For this review, take the finished solid that the model builds, in its own axes (mm). Face numbers are marked on the shaded views. Give positions to 0.01 mm unless a question says otherwise; leave off trailing zeros. Loops run counter-clockwise (first coordinate to the right, second up) from the corner with the lowest first, then second, coordinate; pieces in that order, holes last.
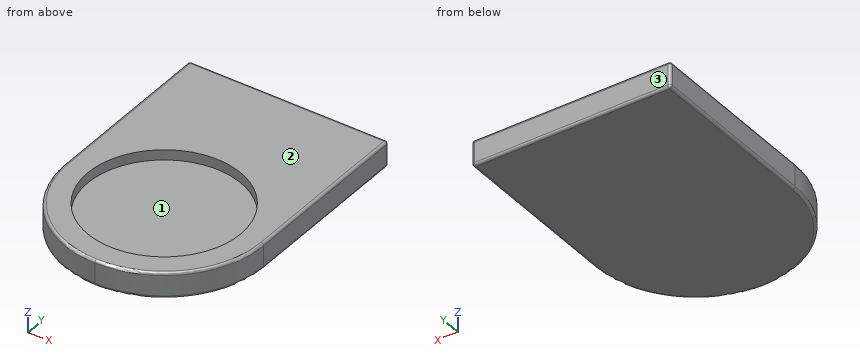
```python
from build123d import *

# Parameters (mm, degrees)
F1_DEPTH = 12.7
F2_DEPTH = 7.62
F3_R     = 1.27


with BuildPart() as f1:
    # F0 (on Top) → F1 (new body)
    with BuildSketch(Plane.XY):
        with BuildLine():
            Line((-49.53, 88.9), (-49.53, 0))
            ThreePointArc((-49.53, 0), (-35.0229988722, -35.0229988722), (0, -49.53))
            Line((0, -49.53), (0, -38.1))
            ThreePointArc((0, -38.1), (-38.1, 0), (0, 38.1))
            Line((0, 38.1), (0, 88.9))
            Line((0, 88.9), (-49.53, 88.9))
        make_face()
        with BuildLine():
            Line((0, -38.1), (0, -49.53))
            ThreePointArc((0, -49.53), (35.0229988722, -35.0229988722), (49.53, 0))
            Line((49.53, 0), (49.53, 88.9))
            Line((49.53, 88.9), (0, 88.9))
            Line((0, 88.9), (0, 38.1))
            ThreePointArc((0, 38.1), (26.9407683632, 26.9407683632), (38.1, 0))
            ThreePointArc((38.1, 0), (26.9407683632, -26.9407683632), (0, -38.1))
        make_face()
    extrude(amount=F1_DEPTH)

    # F0 (on Top) → F2 (join)
    with BuildSketch(Plane.XY):
        with BuildLine():
            ThreePointArc((0, 38.1), (-38.1, 0), (0, -38.1))
            Line((0, -38.1), (0, 38.1))
        make_face()
        with BuildLine():
            Line((0, 38.1), (0, -38.1))
            ThreePointArc((0, -38.1), (26.9407683632, -26.9407683632), (38.1, 0))
            ThreePointArc((38.1, 0), (26.9407683632, 26.9407683632), (0, 38.1))
        make_face()
    extrude(amount=F2_DEPTH)

    # F3
    f3_edges = [f1.edges().sort_by_distance(p)[0] for p in [
        (49.53, 44.45, 12.7),
        (49.53, 88.9, 6.35),
        (0, 88.9, 12.7),
        (0, 88.9, 0),
        (49.53, 44.45, 0),
        (-49.53, 88.9, 6.35),
    ]]
    fillet(f3_edges, radius=F3_R)


solid = f1.part
```
Q1. Consider section A-A on z = 9. Give the boundary of the cut face in (x, y).
Answers:
outline: (-49.53, 0) arc R49.53 ccw to (49.53, 0) - (49.53, 87.63) arc R1.27 ccw to (48.26, 88.9) - (-48.26, 88.9) arc R1.27 ccw to (-49.53, 87.63) - close; hole circle Ø76.2 at (0, 0)
Q2. For pin 1 Ø1 at (y, z) = (-28, 3) entering from -X; pin 2 Ø23 at (x, y) = (4.5, 0.5) entering from +Z; pin 3 Ø1 at (x, z) = (-29, 9) entering from -Y, all flat-tipped, find the tip position at first contact; note any pin that passes through.
Answers:
pin 1: stops at x = -41.19
pin 2: stops at z = 7.62
pin 3: stops at y = -40.51
Q3. Consider section B-B on y = 26. Give the boundary of the cut face in (x, z), plus the area to 3 significant figures.
Answers:
outline: (-49.53, 1.27) arc R1.27 ccw to (-48.26, 0) - (48.26, 0) arc R1.27 ccw to (49.53, 1.27) - (49.53, 11.43) arc R1.27 ccw to (48.26, 12.7) - (27.85, 12.7) - (27.85, 7.62) - (-27.85, 7.62) - (-27.85, 12.7) - (-48.26, 12.7) arc R1.27 ccw to (-49.53, 11.43) - close
area: 974 mm2
Q4. For probe 1 along Y at (x, z) = (-1.5, 9); probe 2 along Z at (x, y) = (-12, -4.5); probe 3 along Y at (x, z) = (-20.5, 9), list the stretches that pass through material, from the lowest coordinate up.
Answers:
probe 1: y = -49.51 to -38.07, 38.07 to 88.9
probe 2: z = 0 to 7.62
probe 3: y = -45.09 to -32.11, 32.11 to 88.9
Q5. Consider section C-C on y = 12. Give the boundary of the cut face in (x, z), plus the area to 3 significant figures.
Answers:
outline: (-49.53, 1.27) arc R1.27 ccw to (-48.26, 0) - (48.26, 0) arc R1.27 ccw to (49.53, 1.27) - (49.53, 11.43) arc R1.27 ccw to (48.26, 12.7) - (36.16, 12.7) - (36.16, 7.62) - (-36.16, 7.62) - (-36.16, 12.7) - (-48.26, 12.7) arc R1.27 ccw to (-49.53, 11.43) - close
area: 889 mm2
Q6. Mouldability with a two-part tool opening along Y and no side actions: class the marked faces 1, 2 and 3 as +Y half, -Y half, draft (parallel to the pull), parting line (faces both ways), or undercut.
Answers:
face 1: undercut
face 2: draft
face 3: +Y half
